Geometry: final body of the model. Coordinates: model frame, mm. A direction names the side the tool comes from. Round coordinates to 2 decimals unless told otherwise and drop trailing zeros. Write each loop counter-clockwise with the first axis right and the second up, starting at its lowest first coordinate (ties: lowest second). Pieces come first, ordered by that corner, then holes. Notation, with made-up numbers: (26, -25) - (37, -25) arc R24 cw to (37, -11) - close; hole circle Ø11 at (72.5, -17.75). An arc over 180 degrees is marked (long way). Write each question's results on one line, items separated by ' | '.
from build123d import *

# Parameters (mm, degrees)
SKETCH1_R               = 13
SKETCH1_R_2             = 4
BOSS_EXTRUDE1_DEPTH     = 45
SKETCH2_W               = 103.301936686
SKETCH2_H               = 74
CUT_EXTRUDE1_DEPTH      = 13.7
CUT_EXTRUDE1_DEPTH_BACK = 64.5


with BuildPart() as part:
    # Sketch1 → Boss-Extrude1 (new body, symmetric)
    with BuildSketch(Plane.XY):
        with BuildLine():
            Line((-28.398063314, 25.4), (-139.7, 25.4))
            Line((-139.7, 25.4), (-139.7, -25.4))
            Line((-139.7, -25.4), (-28.398063314, -25.4))
            ThreePointArc((-28.398063314, -25.4), (38.1, 0), (-28.398063314, 25.4))
        make_face()
        Circle(SKETCH1_R, mode=Mode.SUBTRACT)
        with Locations((-131.7, 0)):
            Circle(SKETCH1_R_2, mode=Mode.SUBTRACT)
        with Locations((-112.7, 0)):
            Circle(SKETCH1_R_2, mode=Mode.SUBTRACT)
        with Locations((-93.7, 0)):
            Circle(SKETCH1_R_2, mode=Mode.SUBTRACT)
        with Locations((-74.7, 0)):
            Circle(SKETCH1_R_2, mode=Mode.SUBTRACT)
        with Locations((-55.7, 0)):
            Circle(SKETCH1_R_2, mode=Mode.SUBTRACT)
    extrude(amount=BOSS_EXTRUDE1_DEPTH, both=True)

    # Sketch2 → Cut-Extrude1 (cut, two sides)
    with BuildSketch(Plane(origin=(0, 25.4, 0), x_dir=(1, 0, 0), z_dir=(0, 1, 0))) as cut_extrude1_sk:
        with Locations((-88.049031657, 0)):
            Rectangle(SKETCH2_W, SKETCH2_H)
    extrude(amount=CUT_EXTRUDE1_DEPTH, mode=Mode.SUBTRACT)
    extrude(cut_extrude1_sk.sketch, amount=-CUT_EXTRUDE1_DEPTH_BACK, mode=Mode.SUBTRACT)


solid = part.part
Q1. Section query C-C, the plane x = -55.7. Return loops of the section in (y, z).
Answer block:
outline: (-25.4, -45) - (-4, -45) - (-4, -37) - (-25.4, -37) - close; (-25.4, 37) - (-4, 37) - (-4, 45) - (-25.4, 45) - close; (4, -45) - (25.4, -45) - (25.4, -37) - (4, -37) - close; (4, 37) - (25.4, 37) - (25.4, 45) - (4, 45) - close
Q2. Pin query (flat end, axial travel): pin 1 (6 mm diameter, centred on x = 10.5, z = 1, fed in from +Y); pin 2 (1.5 mm diameter, centred on y = -11, z = -33.5, fed in from +X); pin 3 (5 mm diameter, centred on x = -74.7, y = 0, fed in from +Z); pin 4 (1.5 mm diameter, centred on y = 28.5, z = -33, fed in from -X). Return the tip coordinate at first contact, or that it passes through.
Answer block:
pin 1: y = 37.35 | pin 2: x = 36.7 | pin 3: through | pin 4: x = -26.11
Q3. Section query D-D, the plane y = 0. Give the number of separate pieces and of enclosed holes in the cut face, plus the area to 3 significant figures.
Answer block:
separate pieces: 12 | enclosed holes: 0 | area: 5,380 mm2
Q4. Mould query, pull axis Z, two halves, no side actions, for faces 1 (the flat face through (-89, 0, -37)), 2 (the flat face through (-52, -8, 45)), 3 (the flat face through (-139.7, 0, -41)). Classes: pulls with the +Z half, pulls with the -Z half, needs draft (parallel to the pull), parting line crosses it, or undercut.
Answer block:
face 1: undercut | face 2: pulls with the +Z half | face 3: needs draft
Q5. Section query B-B, the plane z = -17. Return loops of the section in (x, y), plus the area to 3 significant figures.
Answer block:
outline: (-36.4, -25.4) - (-28.4, -25.4) arc R38.1 ccw (long way) to (-28.4, 25.4) - (-36.4, 25.4) - close; hole circle Ø26 at (0, 0) | area: 4,100 mm2
Q6. Access query for faces 4 (the flat face through (-35, -25.4, -6)), 5 (the flat face through (-89, 0, 37)), 6 (the cylindrical face through (-97.696, 0.176, -41.056)), 7 (the flat face through (-52, -8, -45)), 8 (the flat face through (-34, 25.4, -3)). Directions: +Z, -Z, +X, -X, +Y, -Y. A direction counts if a zero-diameter tool reaches every point of the face in a straight line with its end or side. Return the directions, or none.
Answer block:
face 4: +Z, -Z, -X, -Y | face 5: -X, +Y, -Y | face 6: +Z, -Z | face 7: -Z, +X, -X, +Y, -Y | face 8: +Z, -Z, -X, +Y
Q7. Section query A-A, the plane x = 0. Return loops of the section in (y, z), plus the area to 3 significant figures.
Answer block:
outline: (-38.1, -45) - (-13, -45) - (-13, 45) - (-38.1, 45) - close; (13, -45) - (38.1, -45) - (38.1, 45) - (13, 45) - close | area: 4,520 mm2
Q8. Ray query, line 1 along Y through (x, z) = (-74.7, 41.25); line 2 along Y through (x, z) = (0, -1.5); line 3 along Z through (x, y) = (-58, 16.5). Return the intervals inside material, ascending.
Answer block:
line 1: -25.4 to -4, 4 to 25.4 | line 2: -38.1 to -13, 13 to 38.1 | line 3: -45 to -37, 37 to 45
